Build history of the part. All positions in model axes, mm. Round coordinates to 2 decimals unless told otherwise and drop trailing zeros. Loops run counter-clockwise (first coordinate to the right, second up) from the corner with the lowest first, then second, coordinate; pieces in that order, holes last. Notation, with made-up numbers: (-4, 61.5) -> (44, 61.5) arc R16 cw to (44, 69.5) -> close; hole circle Ø6 at (26.25, -26). An arc over 180 degrees is marked (long way). Put each result on its own line as item: value. Start each with the question number.
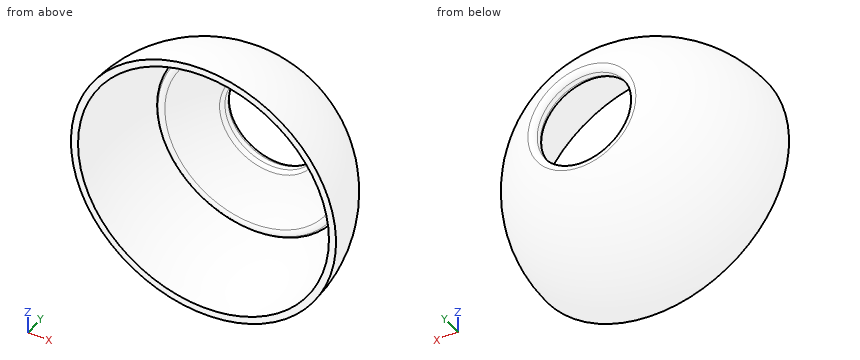
```python
from build123d import *

# Parameters (mm, degrees)
CROQUIS2_W            = 10
CROQUIS2_H            = 14
REDONDEO1_R           = 1
CROQUIS3_R            = 29.845650159
CORTAR_EXTRUIR1_DEPTH = 30


with BuildPart() as part:
    # Croquis1 → Revolución3 (revolve)
    with BuildSketch(Plane(origin=(0, 0, 0), x_dir=(0, 0, -1), z_dir=(1, 0, 0))):
        with BuildLine():
            Line((-0.5, 27.995535358), (-0.5, 26.495282599))
            Line((-0.5, 26.495282599), (-0.5, 24.9949995))
            ThreePointArc((-0.5, 24.9949995), (-10.791516482, 22.5509018), (-19.151111078, 16.069690242))
            Line((-19.151111078, 16.069690242), (-20.300177743, 17.033871657))
            ThreePointArc((-20.300177743, 17.033871657), (-24.017156356, -11.199383936), (0, -26.5))
            Line((0, -26.5), (0, -28))
            ThreePointArc((0, -28), (-27.998883817, -0.250009966), (-0.5, 27.995535358))
        make_face()
    revolve(axis=Axis((0, 29, 0), (0, -1, 0)))

    # Croquis2 → Cortar-Revolución2 (revolve, cut)
    with BuildSketch(Plane(origin=(0, 0, 0), x_dir=(0, 0, -1), z_dir=(1, 0, 0))):
        with Locations((-5, 23)):
            Rectangle(CROQUIS2_W, CROQUIS2_H)
    revolve(axis=Axis((0, 0, 0), (0, 1, 0)), mode=Mode.SUBTRACT)

    # Redondeo1
    redondeo1_edges = [part.edges().sort_by_distance(p)[0] for p in [
        (0, 22.912878475, -10),
        (0, 26.153393661, -10),
        (0, 16.069690242, -19.151111078),
    ]]
    fillet(redondeo1_edges, radius=REDONDEO1_R)

    # Croquis3 → Cortar-Extruir1 (cut)
    with BuildSketch(Plane(origin=(0, 0, 0), x_dir=(1, 0, 0), z_dir=(0, 1, 0))):
        Circle(CROQUIS3_R)
    extrude(amount=-CORTAR_EXTRUIR1_DEPTH, mode=Mode.SUBTRACT)


solid = part.part
```
Item 1: Cut at A-A on y = 21.75. Write the cut outline in (x, z).
Item 2: Drop flat-ended pins along their axis: pin 1 (1 mm diameter, centred on y = 15, z = 16.5, fed in from +X); pin 2 (3 mm diameter, centred on x = -0.5, y = 14, fed in from -Z); pin 3 (8 mm diameter, centred on x = 8, z = 17.5, fed in from -Y); pin 4 (12 mm diameter, centred on x = 22, z = -5.5, fed in from -Y). Give the stop position or say it passes through.
Item 3: Cut at C-C on y = 11.5. Write the cut outline in (x, z), then the cut area to 3 significant figures.
Item 4: Wall check: line 1 (X direction, y = 24.4, z = 0); line 2 (X direction, y = 15, z = -1); line 3 (Z direction, x = -3.5, y = 6.5). Give the ranges that are in metal, low to high. Write a range as from..to.
Item 5: Cut at B-B on z = 22. Write the cut outline in (x, y).
Ans:
1. outline: circle Ø35.27 at (0, 0); hole circle Ø24.65 at (0, 0)
2. pin 1: stops at x = 17.57
2. pin 2: stops at z = -25.05
2. pin 3: stops at y = 12.73
2. pin 4: stops at y = 0
3. outline: circle Ø51.06 at (0, 0); hole circle Ø47.75 at (0, 0)
3. area: 257 mm2
4. line 1: x = -13.73..-10, 10..13.73
4. line 2: x = -23.62..-21.82, 21.82..23.62
4. line 3: z = -27.01..-25.45, 25.45..27.01
5. outline: (-17.32, 0) -> (-14.77, 0) arc R14.77 cw to (14.77, 0) -> (17.32, 0) arc R17.32 ccw to start
